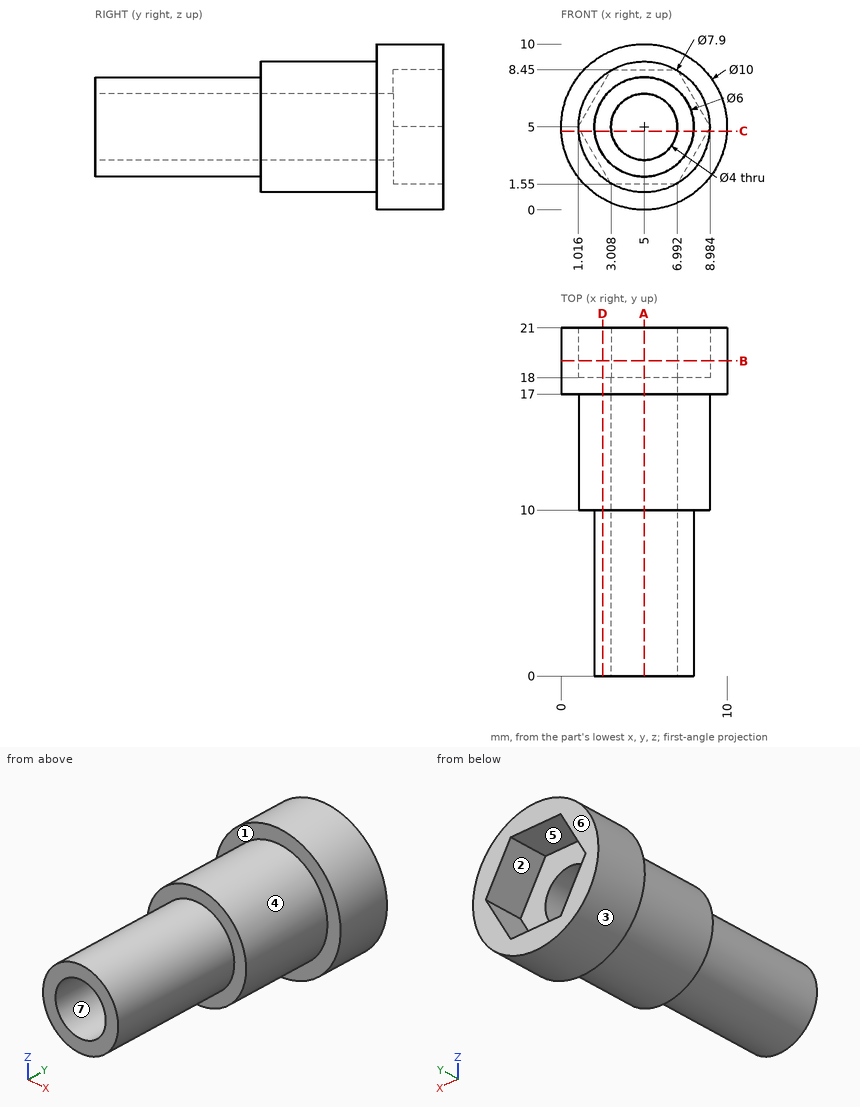
Could you check a few things on this drawing? It's one solid part, dimensions in mm from its lowest x, y, z. A direction names the side the tool comes from. Give positions to 0.01 mm unless a question says otherwise; leave off trailing zeros. Loops run counter-clockwise (first coordinate to the right, second up) from the corner with the lowest first, then second, coordinate; pieces in that order, holes last. Notation, with made-up numbers: M 13.5,45 L 61.5,45 A30 cw 61.5,70 Z; hole C 62.5,48 d2. An arc over 180 degrees is marked long. One line per question, with ' | ' between items. Start each with the question number.
Q1. If we section it at C-C (z = 4.75): Please give me the cut outline in (x, y).
Q2. For the marked faces 1, 2 and 3, which set-ups out of +Z, -Z, +X, -X, +Y, -Y let a thin tool reach every point of the face, with its end or its side?
Q3. If we section it at A-A (x = 5): Please give me the cut outline in (y, z).
Q4. If we section it at D-D (x = 2.5): Please give me the cut outline in (y, z), plus the area to 3 significant figures.
Q5. If we section it at B-B (y = 19): Please give me the cut outline in (x, z).
Q6. If we mould it in two halves opening along X, with no side actions, what happens to the marked faces 4, 5, 6 and 7? For each: +X half, -X half, draft (parallel to the pull), parting line (faces both ways), or undercut.
Q7. If I drill on line 1 (Z direction, x = 5, y = 9.25); line 2 (Y direction, x = 6.25, z = 1.5), over which ranges is the centre line in solid material (lowest first)? Write a range as from..to.
Q8. For pin 1 Ø6 at (y, z) = (3, 1.5) entering from -X; pin 2 Ø3 at (x, z) = (5, 5) entering from -Y; pin 3 Ø1 at (y, z) = (8, 2) entering from +X; pin 4 Ø3 at (x, z) = (6, 5) entering from +Y, each with a flat end and sliding along its axis, tell me the tip position at first contact or that it passes through.
Computed:
1) outline: M 0.01,17 L 1.06,17 L 1.06,10 L 2.01,10 L 2.01,0 L 3.02,0 L 3.02,18 L 1.16,18 L 1.16,21 L 0.01,21 Z; M 6.98,0 L 7.99,0 L 7.99,10 L 8.94,10 L 8.94,17 L 9.99,17 L 9.99,21 L 8.84,21 L 8.84,18 L 6.98,18 Z
2) face 1: -Y | face 2: +Y | face 3: +Y, -Y
3) outline: M 0,2 L 10,2 L 10,1.05 L 17,1.05 L 17,0 L 21,0 L 21,1.55 L 18,1.55 L 18,3 L 0,3 Z; M 0,7 L 18,7 L 18,8.45 L 21,8.45 L 21,10 L 17,10 L 17,8.95 L 10,8.95 L 10,8 L 0,8 Z
4) outline: M 0,3.34 L 10,3.34 L 10,1.94 L 17,1.94 L 17,0.67 L 21,0.67 L 21,2.43 L 18,2.43 L 18,7.57 L 21,7.57 L 21,9.33 L 17,9.33 L 17,8.06 L 10,8.06 L 10,6.66 L 0,6.66 Z | area: 95.2 mm²
5) outline: C 5,5 d10; hole M 1.02,5 L 3.01,1.55 L 6.99,1.55 L 8.98,5 L 6.99,8.45 L 3.01,8.45 Z
6) face 4: parting line | face 5: undercut | face 6: draft | face 7: undercut
7) line 1: z = 2..3, 7..8 | line 2: y = 10..21
8) pin 1: stops at x = 2.04 | pin 2: passes through | pin 3: stops at x = 6.66 | pin 4: stops at y = 18
